from build123d import *

# Parameters (mm, degrees)
F0_R     = 3
F1_DEPTH = 3
F2_SIZE  = 1
F3_SIZE  = 2


with BuildPart() as f1:
    # F0 (on Front) → F1 (new body)
    with BuildSketch(Plane.XZ):
        with BuildLine():
            ThreePointArc((5, 0), (15, -10), (25, 0))
            ThreePointArc((25, 0), (0, 25), (-25, 0))
            ThreePointArc((-25, 0), (-23.826115, -4.701031), (-20.580062, -8.298368))
            Line((-20.580062, -8.298368), (-17.955888, -10.062938))
            ThreePointArc((-17.955888, -10.062938), (-13.137419, -14.846001), (-10.433443, -21.073669))
            Line((-10.433443, -21.073669), (-10.024779, -22.902048))
            ThreePointArc((-10.024779, -22.902048), (-10.075894, -22.879606), (-10.126959, -22.857049))
            Line((-10.126959, -22.857049), (-5.949267, -54.778603))
            ThreePointArc((-5.949267, -54.778603), (-3.957801, -58.509524), (0, -60))
            Line((0, -60), (0, -57))
            Line((0, -57), (0, -5))
            ThreePointArc((0, -5), (-3.535534, 3.535534), (5, 0))
        make_face()
        with Locations((-15, 0)):
            Circle(F0_R, mode=Mode.SUBTRACT)
        with Locations((15, 0)):
            Circle(F0_R, mode=Mode.SUBTRACT)
        with BuildLine():
            Line((-10.024779, -22.902048), (-10.433443, -21.073669))
            ThreePointArc((-10.433443, -21.073669), (-10.274972, -21.865774), (-10.152199, -22.664192))
            Line((-10.152199, -22.664192), (-10.126959, -22.857049))
            ThreePointArc((-10.126959, -22.857049), (-10.075894, -22.879606), (-10.024779, -22.902048))
        make_face()
        with BuildLine():
            Line((-10.126959, -22.857049), (-10.152199, -22.664192))
            ThreePointArc((-10.152199, -22.664192), (-10.139879, -22.760341), (-10.128077, -22.856554))
            ThreePointArc((-10.128077, -22.856554), (-10.127518, -22.856802), (-10.126959, -22.857049))
        make_face()
    extrude(amount=F1_DEPTH)

    # F2
    f2_edges = [f1.edges().sort_by_distance(p)[0] for p in [
        (-18, -3, 0),
        (12, -3, 0),
    ]]
    chamfer(f2_edges, length=F2_SIZE)

    # F3
    f3_edges = [f1.edges().sort_by_distance(p)[0] for p in [
        (0, -3, -32.5),
    ]]
    chamfer(f3_edges, length=F3_SIZE)


solid = f1.part
Design review of the part built by this model. Coordinates are the model's own, in mm. Coordinates: 2 decimals unless noted, no trailing zeros. Loops run counter-clockwise (first coordinate to the right, second up) from the corner with the lowest first, then second, coordinate; pieces in that order, holes last. Notation, with made-up numbers: (79, 29.25) -> (120, 29.25) arc R13 cw to (120, 39.25) -> close; hole circle Ø2 at (34.5, 75). An arc over 180 degrees is marked (long way). Use a Markdown table: item, result. Add a question column.
Item 1: We need section C-C, the plane x = -15. Write out the cut boundary in (y, z), and give its area (3 significant figures).
Item 2: The part is to be moulded in two halves that separate along X. For faces 1 (the flat face through (-6, -3, 2)), 2 (the cylindrical face through (15, -1, -10)), 3 (the cylindrical face through (-10.277, -1.479, -21.855)), say which applies: +X half, -X half, draft (parallel to the pull), parting line (faces both ways), or undercut.
Item 3: We need section D-D, the plane x = 8. Write out the cut boundary in (y, z), and give its area (3 significant figures).
Item 4: We need section A-A, the plane x = 15. Write out the cut boundary in (y, z), and give its area (3 significant figures).
Item 5: We need section B-B, the plane z = 1. Count the separate pieces of the cut face and the enclosed holes in it, and give its area (3 significant figures).
Item 6: Clearance check with a flat-ended pin moving along its axis: P1, Ø0.5, axis at y = -0.5, z = -34.5, coming from the +X side. State where the tip first meets the part, or that it passes through.
Item 7: Wall thickness on L1, parallel to Z at x = -1.5, y = -0.6; L2, parallel to Z at x = 14.5, y = -2.35; L3, parallel to Z at x = 0, y = -1.25: over which ranges is each line inside the solid? List them lowest first. Write a range as from..to.
Numbers:
| question | item | result |
|---|---|---|
| 1 | outline | (-3, -12.55) -> (0, -12.55) -> (0, -3) -> (-2, -3) -> (-3, -4) -> close; (-3, 4) -> (-2, 3) -> (0, 3) -> (0, 20) -> (-3, 20) -> close |
| 1 | area | 78.7 mm^2 |
| 2 | face 1 | draft |
| 2 | face 2 | undercut |
| 2 | face 3 | -X half |
| 3 | outline | (-3, -7.14) -> (0, -7.14) -> (0, 23.69) -> (-3, 23.69) -> close |
| 3 | area | 92.5 mm^2 |
| 4 | outline | (-3, -10) -> (0, -10) -> (0, -3) -> (-2, -3) -> (-3, -4) -> close; (-3, 4) -> (-2, 3) -> (0, 3) -> (0, 20) -> (-3, 20) -> close |
| 4 | area | 71.0 mm^2 |
| 5 | separate pieces | 4 |
| 5 | enclosed holes | 0 |
| 5 | area | 84.4 mm^2 |
| 6 | P1 | stops at x = 0 |
| 7 | L1 | z = -59.81..-4.77, 4.77..24.95 |
| 7 | L2 | z = -9.99..-3.31, 3.31..20.37 |
| 7 | L3 | z = 5..25 |
